from build123d import *

# Parameters (mm, degrees)
IZIM1_R                     = 60
Y_KSEKLIK_EKSTR_ZYON1_DEPTH = 200
IZIM2_R                     = 100
Y_KSEKLIK_EKSTR_ZYON2_DEPTH = 300
IZIM3_R                     = 60
Y_KSEKLIK_EKSTR_ZYON3_DEPTH = 200
KES_EKSTR_ZYON1_DEPTH       = 200


with BuildPart() as part:
    # Çizim1 → Yükseklik-Ekstrüzyon1 (new body)
    with BuildSketch(Plane(origin=(0, 0, 0), x_dir=(0, 0, -1), z_dir=(1, 0, 0))):
        Circle(IZIM1_R)
    extrude(amount=Y_KSEKLIK_EKSTR_ZYON1_DEPTH)

    # Çizim2 → Yükseklik-Ekstrüzyon2 (add)
    with BuildSketch(Plane(origin=(200, 0, 0), x_dir=(0, 0, -1), z_dir=(1, 0, 0))):
        Circle(IZIM2_R)
    extrude(amount=Y_KSEKLIK_EKSTR_ZYON2_DEPTH)

    # Çizim3 → Yükseklik-Ekstrüzyon3 (add)
    with BuildSketch(Plane(origin=(500, 0, 0), x_dir=(0, 0, -1), z_dir=(1, 0, 0))):
        Circle(IZIM3_R)
    extrude(amount=Y_KSEKLIK_EKSTR_ZYON3_DEPTH)

    # Çizim4 → Kes-Ekstrüzyon1 (cut)
    with BuildSketch(Plane(origin=(0, 50, 0), x_dir=(1, 0, 0), z_dir=(0, 1, 0))):
        with BuildLine():
            Line((250, 25), (450, 25))
            ThreePointArc((450, 25), (475, 0), (450, -25))
            Line((450, -25), (250, -25))
            ThreePointArc((250, -25), (225, 0), (250, 25))
        make_face()
    extrude(amount=KES_EKSTR_ZYON1_DEPTH, mode=Mode.SUBTRACT)


solid = part.part
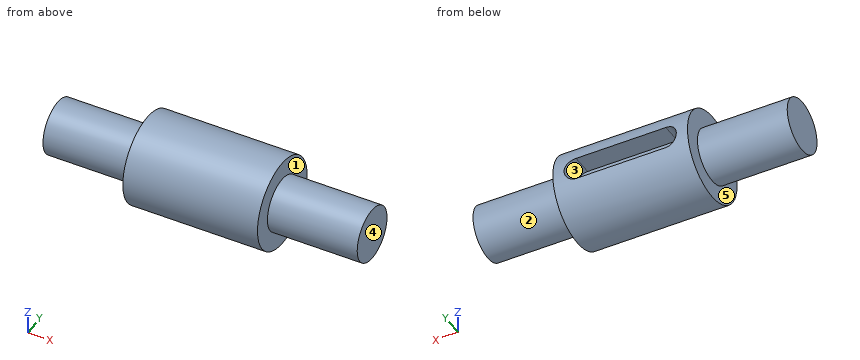
Here's how the part is built. I have some questions about the finished solid (model axes, mm). Face numbers are marked on the shaded views. A direction names the side the tool comes from. Give positions to 0.01 mm unless a question says otherwise; leave off trailing zeros. Order: outer loops, then holes, each group sorted by start corner. A loop starts at its lowest first (then second) coordinate and runs counter-clockwise, first axis right, second up. Notation, with made-up numbers: (23, -22) -> (34, -22) arc R10 cw to (34, -3) -> close; hole circle Ø8 at (79, 57.25). An arc over 180 degrees is marked (long way). Use a Markdown table: item, result. Add a question column.
Item 1: Imagine slicing it at C-C on y = 70. Please give me the cut outline in (x, z), plus the area to 3 significant figures.
Item 2: Imagine slicing it at B-B on z = 51. Please give me the cut outline in (x, y), plus the area to 3 significant figures.
Item 3: Imagine slicing it at A-A on y = 38. Please give me the cut outline in (x, z), plus the area to 3 significant figures.
Item 4: Imagine slicing it at D-D on x = 481.5. Please give me the cut outline in (y, z), plus the area to 3 significant figures.
Item 5: Will these pins go through, and if not, where does the flat tip stop? pin 1 (1.5 mm diameter, centred on y = 15, z = 14.5, fed in from -X); pin 2 (6 mm diameter, centred on x = 237, y = 41.5, fed in from -Z); pin 3 (14 mm diameter, centred on x = 311.5, y = 83, fed in from -Z); pin 4 (5 mm diameter, centred on y = -37.5, z = -67, fed in from +X).
Item 6: For the marked faces 4 and 5, which set-ups out of +Z, -Z, +X, -X, +Y, -Y let a thin tool reach every point of the face, with its end or its side?
Item 7: If we mould it in two halves opening along Z, with no side actions, what happens to the marked faces 1, 2 and 3? For each: pulls with the +Z half, pulls with the -Z half, needs draft (parallel to the pull), parting line crosses it, or undercut.
Item 8: I need wall thicknesses on line 1 (X direction, y = 24.5, z = -69); line 2 (Y direction, x = 317, z = -2.5); line 3 (Z direction, x = 450, y = 79). Which ranges of each line are inside material? Lowest first, please.
Data:
| question | item | result |
|---|---|---|
| 1 | outline | (200, -71.41) -> (500, -71.41) -> (500, 71.41) -> (200, 71.41) -> close; hole (250, -25) -> (450, -25) arc R25 ccw to (450, 25) -> (250, 25) arc R25 ccw to start |
| 1 | area | 30,900 mm² |
| 2 | outline | (0, -31.61) -> (200, -31.61) -> (200, -86.02) -> (500, -86.02) -> (500, -31.61) -> (700, -31.61) -> (700, 31.61) -> (500, 31.61) -> (500, 86.02) -> (200, 86.02) -> (200, 31.61) -> (0, 31.61) -> close |
| 2 | area | 76,900 mm² |
| 3 | outline | (0, -46.43) -> (200, -46.43) -> (200, -92.5) -> (500, -92.5) -> (500, -46.43) -> (700, -46.43) -> (700, 46.43) -> (500, 46.43) -> (500, 92.5) -> (200, 92.5) -> (200, 46.43) -> (0, 46.43) -> close |
| 3 | area | 92,600 mm² |
| 4 | outline | circle Ø200 at (0, 0) |
| 4 | area | 31,400 mm² |
| 5 | pin 1 | stops at x = 0 |
| 5 | pin 2 | stops at z = -92.29 |
| 5 | pin 3 | stops at z = -64.99 |
| 5 | pin 4 | stops at x = 500 |
| 6 | face 4 | +Z, -Z, +X, +Y, -Y |
| 6 | face 5 | -X |
| 7 | face 1 | needs draft |
| 7 | face 2 | parting line crosses it |
| 7 | face 3 | undercut |
| 8 | line 1 | x = 200 to 500 |
| 8 | line 2 | y = -99.97 to 50 |
| 8 | line 3 | z = -61.31 to -25, 25 to 61.31 |
